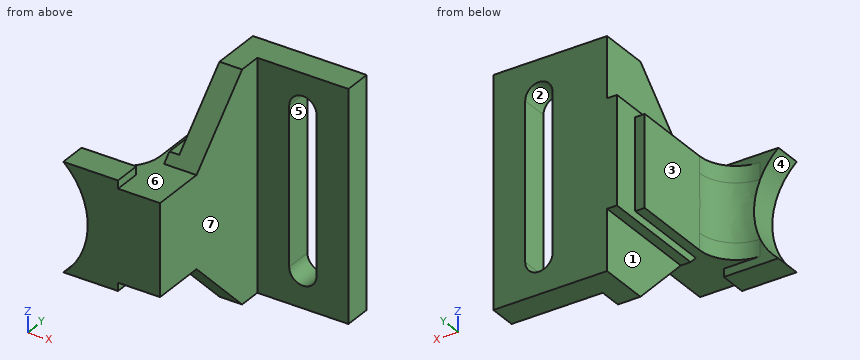
```python
from build123d import *

# Parameters (mm, degrees)
SKETCH1_R               = 1.5
BOSS_EXTRUDE1_DEPTH     = 3
SKETCH3_W               = 4.615398666
SKETCH3_H               = 10
BOSS_EXTRUDE2_DEPTH     = 12.9997796
FILLET7_R               = 1
CUT_EXTRUDE4_DEPTH      = 10
SKETCH9_W               = 13.564457496
SKETCH9_H               = 25
SKETCH9_R               = 1.5
BOSS_EXTRUDE3_DEPTH     = 3
CHAMFER1_SIZE           = 10
CHAMFER2_SIZE           = 10
FILLET8_R               = 4
CUT_EXTRUDE5_DEPTH      = 27.880201216
CUT_EXTRUDE5_DEPTH_BACK = 27.880201216
SKETCH10_W              = 8.131195533
SKETCH10_H              = 6.749631571
SKETCH10_H_2            = 7.013496214
CUT_EXTRUDE6_DEPTH      = 10


with BuildPart() as part:
    # Sketch1 → Boss-Extrude1 (new body)
    with BuildSketch(Plane(origin=(0, 0, 0), x_dir=(1, 0, 0), z_dir=(0, 1, 0))):
        Polygon((-3, -11.32792047), (3, -11.32792047), (3, -5), (7.615398666, -5), (7.615398666, 5), (3, 5), (3, 11.32792047), (-3, 11.32792047), align=None)
        with Locations(Location((0, 8.5, 0), (0, 0, 270))):
            Circle(SKETCH1_R, mode=Mode.SUBTRACT)
        with Locations(Location((0, -8.5, 0), (0, 0, 270))):
            Circle(SKETCH1_R, mode=Mode.SUBTRACT)
    extrude(amount=BOSS_EXTRUDE1_DEPTH)

    # Sketch3 → Boss-Extrude2 (add)
    with BuildSketch(Plane(origin=(0, 3, 0), x_dir=(1, 0, 0), z_dir=(0, 1, 0))):
        with Locations((5.307699333, 0)):
            Rectangle(SKETCH3_W, SKETCH3_H)
    extrude(amount=BOSS_EXTRUDE2_DEPTH)

    # Fillet7
    fillet7_edges = [part.edges().sort_by_distance(p)[0] for p in [
        (3, 1.5, 11.32792047),
        (3, 1.5, -11.32792047),
    ]]
    fillet(fillet7_edges, radius=FILLET7_R)

    # Sketch7 → Cut-Extrude4 (cut)
    with BuildSketch(Plane.XZ):
        with BuildLine():
            Line((-3.65526474, -6.392053518), (-3.78188192, 6.478485425))
            ThreePointArc((-3.78188192, 6.478485425), (-0.319780446, 0.076652438), (-3.65526474, -6.392053518))
        make_face()
    extrude(amount=-CUT_EXTRUDE4_DEPTH, mode=Mode.SUBTRACT)

    # Sketch9 → Boss-Extrude3 (add)
    with BuildSketch(Plane(origin=(0, 15.9997796, 0), x_dir=(1, 0, 0), z_dir=(0, 1, 0))):
        with Locations((10.833169918, 0)):
            Rectangle(SKETCH9_W, SKETCH9_H)
        with Locations(Location((12.615398666, 6, 0), (0, 0, 270))):
            Circle(SKETCH9_R, mode=Mode.SUBTRACT)
        with Locations(Location((12.615398666, -6, 0), (0, 0, 270))):
            Circle(SKETCH9_R, mode=Mode.SUBTRACT)
    extrude(amount=BOSS_EXTRUDE3_DEPTH)

    # Chamfer1
    # the kernel refuses this chamfer: 10 mm, written as the material it adds along each edge
    with BuildSketch(Plane(origin=(4.05094117, 15.9997796, 5), x_dir=(0, -0.9996219169112968, -0.027495876610586403), z_dir=(1, 0, 0))) as chamfer1_piece_1_section:
        Polygon((CHAMFER1_SIZE * 0.999621916911, -CHAMFER1_SIZE * 0.0274958766106), (-CHAMFER1_SIZE * 0.0274958766106, -CHAMFER1_SIZE * 0.999621916911), (0, 0), align=None)
    chamfer1_piece_1 = extrude(amount=3.564457497, mode=Mode.PRIVATE)
    chamfer1_piece_1 = split(chamfer1_piece_1, bisect_by=Plane(origin=(5.833169918, 12.4997796, 12.5), z_dir=(0, 0, -1)), keep=Keep.TOP, mode=Mode.PRIVATE)
    add(chamfer1_piece_1)

    # Chamfer2
    # the kernel refuses this chamfer: 10 mm, written as the material it adds along each edge
    with BuildSketch(Plane(origin=(7.615398666, 15.9997796, -5), x_dir=(0, -0.9996219169112968, 0.027495876610586403), z_dir=(-1, 0, 0))) as chamfer2_piece_1_section:
        Polygon((CHAMFER2_SIZE * 0.999621916911, -CHAMFER2_SIZE * 0.0274958766106), (-CHAMFER2_SIZE * 0.0274958766106, -CHAMFER2_SIZE * 0.999621916911), (0, 0), align=None)
    chamfer2_piece_1 = extrude(amount=3.564457497, mode=Mode.PRIVATE)
    chamfer2_piece_1 = split(chamfer2_piece_1, bisect_by=Plane(origin=(5.833169918, 12.4997796, -12.5), z_dir=(0, 0, 1)), keep=Keep.TOP, mode=Mode.PRIVATE)
    add(chamfer2_piece_1)

    # Fillet8
    fillet8_edges = [part.edges().sort_by_distance(p)[0] for p in [
        (3, 3, 0),
    ]]
    fillet(fillet8_edges, radius=FILLET8_R)

    # Sketch10 → Cut-Extrude5 (cut, two sides: drawn at the far end of the back side and taken through both)
    with BuildSketch(Plane(origin=(0, 3, 0), x_dir=(1, 0, 0), z_dir=(0, 1, 0)).offset(-CUT_EXTRUDE5_DEPTH_BACK)):
        with Locations((1.065597767, 9.256059268)):
            Rectangle(SKETCH10_W, SKETCH10_H)
        with Locations((1.065597767, -9.38799159)):
            Rectangle(SKETCH10_W, SKETCH10_H_2)
    extrude(amount=CUT_EXTRUDE5_DEPTH + CUT_EXTRUDE5_DEPTH_BACK, mode=Mode.SUBTRACT)

    # Sketch11 → Cut-Extrude6 (cut)
    with BuildSketch(Plane(origin=(0, 18.9997796, 0), x_dir=(1, 0, 0), z_dir=(0, 1, 0))):
        with BuildLine():
            Line((14.115398666, 8.584889461), (14.115398666, -8.584889461))
            ThreePointArc((14.115398666, -8.584889461), (12.615398666, -10.084889461), (11.115398666, -8.584889461))
            Line((11.115398666, -8.584889461), (11.115398666, 8.584889461))
            ThreePointArc((11.115398666, 8.584889461), (12.615398666, 10.084889461), (14.115398666, 8.584889461))
        make_face()
    extrude(amount=-CUT_EXTRUDE6_DEPTH, mode=Mode.SUBTRACT)


solid = part.part
```
Model file for the job. Use its own axes, mm. Face numbers are marked on the shaded views. A direction names the side the tool comes from. Coordinates: 2 decimals unless noted, no trailing zeros. Loops run counter-clockwise (first coordinate to the right, second up) from the corner with the lowest first, then second, coordinate; pieces in that order, holes last. Notation, with made-up numbers: (-26, 45) - (20, 45) arc R30 ccw to (20, 72) - close; hole circle Ø2 at (3, 41). An arc over 180 degrees is marked (long way). Answer as a JSON object with one key per item and string values. Group by question number.
(1) Probe line 1 along X through (y, z) = (17.5, -5); line 2 along X through (y, z) = (15, -3); line 3 along Z through (x, y) = (4, 3.5). List the from-to ranges inside material, lowest first.
(2) Cut at C-C (y = 2.25). Give the cut face in (x, z), then the cut area to 3 significant figures.
(3) Cut at B-B (x = 5.5). Give the cut face in (y, z).
(4) Flat gauge pins, fed straight in: pin 1 (0.9 mm diameter, centred on x = 4.5, y = 12.5, fed in from -Z); pin 2 (8 mm diameter, centred on x = 10.5, y = 6, fed in from -Z); pin 3 (9.5 mm diameter, centred on x = 5.5, y = 6.5, fed in from -Z); pin 4 (1.5 mm diameter, centred on x = -0.5, z = -2.5, fed in from -Y). Where does each tip first touch, or does it go through?
(5) Cut at A-A (y = 16.5). Give the cut face in (x, z), then the cut area to 3 significant figures.
(6) Two-plate mould, pull along X, no slides. Class the marked faces 4, 5, 6 and 7: released by +X, released by -X, zero draft, split by the parting line, or undercut.
(7) Tool access for the marked faces 1, 2 and 3: list every direction of +Z, -Z, +X, -X, +Y, -Y with a clear straight run to the whole face (end or side of a thin tool).
(8) Cut at D-D (z = -9.75). Give the cut face in (x, y).
Geometry says:
{
 "1": {"line 1": "x = 4.05 to 11.12, 14.12 to 17.62", "line 2": "x = 3 to 7.62", "line 3": "z = -5 to 5"},
 "2": {"outline": "(-3, -5.88) - (3, -5.88) - (3, -5) - (7.62, -5) - (7.62, 5) - (3, 5) - (3, 5.88) - (-3, 5.88) arc R7.79 cw to start", "area": "94.9 mm^2"},
 "3": {"outline": "(0, -5) - (6, -5) - (13.5, -12.5) - (19, -12.5) - (19, 12.5) - (13.5, 12.5) - (6, 5) - (0, 5) - close"},
 "4": {"pin 1": "stops at z = -5.88", "pin 2": "stops at z = -7.77", "pin 3": "stops at z = -10.25", "pin 4": "stops at y = 0"},
 "5": {"outline": "(4.05, -5.88) - (5.13, -5.88) - (5.13, -12.5) - (17.62, -12.5) - (17.62, 12.5) - (5.13, 12.5) - (5.13, 5.88) - (4.05, 5.88) - close; hole (11.12, -8.58) arc R1.5 ccw to (14.12, -8.58) - (14.12, 8.58) arc R1.5 ccw to (11.12, 8.58) - close", "area": "266 mm^2"},
 "6": {"face 4": "released by -X", "face 5": "undercut", "face 6": "zero draft", "face 7": "released by +X"},
 "7": {"face 1": "-Z, -X, +Y, -Y", "face 2": "+Y, -Y", "face 3": "+Z, -Z, -X, +Y"},
 "8": {"outline": "(5.13, 10.75) - (7.62, 10.75) - (7.62, 16) - (11.67, 16) - (11.67, 19) - (5.13, 19) - close; (13.56, 16) - (17.62, 16) - (17.62, 19) - (13.56, 19) - close"}
}
